```python
from build123d import *

# Parameters (mm, degrees)
SKETCH_1_W      = 2
SKETCH_1_H      = 12
EXTRUDE_1_DEPTH = 2.9
EXTRUDE_START   = -2
SKETCH_2_W      = 3.3
SKETCH_2_H      = 1.5
SKETCH_2_H_2    = 1.8
EXTRUDE_2_DEPTH = 5
SKETCH_3_W      = 10.525
SKETCH_3_H      = 2.9
EXTRUDE_3_DEPTH = 2
EXTRUDE_START_2 = -2.9
SKETCH_5_W      = 5
SKETCH_5_H      = 1
EXTRUDE_5_DEPTH = 17.8


with BuildPart() as part:
    # 草图1 → 凸台-拉伸1 (new body)
    with BuildSketch(Plane(origin=(0, 0, 0), x_dir=(1, 0, 0), z_dir=(0, 1, 0))):
        Rectangle(SKETCH_1_W, SKETCH_1_H)
    extrude(amount=EXTRUDE_1_DEPTH)

    # 草图2 → 凸台-拉伸2 (add)
    with BuildSketch(Plane(origin=(1, 0, 0), x_dir=(0, 0, -1), z_dir=(1, 0, 0)).offset(EXTRUDE_START)):
        with Locations((4.35, 3.25)):
            Rectangle(SKETCH_2_W, SKETCH_2_H)
        with Locations((4.35, -0.2)):
            Rectangle(SKETCH_2_W, SKETCH_2_H_2)
    extrude(amount=EXTRUDE_2_DEPTH)

    # 草图3 → 凸台-拉伸3 (add)
    with BuildSketch(Plane.ZY.offset(1)):
        with Locations((2.5625, 1.45)):
            Rectangle(SKETCH_3_W, SKETCH_3_H)
    extrude(amount=-EXTRUDE_3_DEPTH)

    # 草图5 → 凸台-拉伸5 (add)
    with BuildSketch(Plane(origin=(0, 2.9, 0), x_dir=(1, 0, 0), z_dir=(0, 1, 0)).offset(EXTRUDE_START_2)):
        with Locations((1.5, -7.325)):
            Rectangle(SKETCH_5_W, SKETCH_5_H)
        with Locations((1.5, -8.325)):
            Rectangle(SKETCH_5_W, SKETCH_5_H)
    extrude(amount=EXTRUDE_5_DEPTH)


solid = part.part
```
Can you work these out from the model? Positions are in its coordinate system, mm. A direction names the side the tool comes from. Coordinates: 2 decimals unless noted, no trailing zeros. Write each loop counter-clockwise with the first axis right and the second up, starting at its lowest first coordinate (ties: lowest second). Pieces come first, ordered by that corner, then holes. Notation, with made-up numbers: M 65,87 L 120,87 A19 cw 120,115 Z; hole C 63,-5.75 d6. An arc over 180 degrees is marked long. Write item = value, one per line. Start each with the question number.
Q1. If I drill on L1, parallel to Y at x = 2, z = -4; L2, parallel to Z at x = 2.8, y = 8.5 (3 decimals); L3, parallel to Y at x = 0, z = 2.25, over which ranges is the centre line in solid material (lowest first)? Write a range as [from, to].
Q2. I'm going to push flat-ended pins straight in: pin 1 (1.6 mm diameter, centred on x = 2.5, z = -3.5, fed in from +Y); pin 2 (0.9 mm diameter, centred on y = 2, z = 1.5, fed in from +X); pin 3 (8 mm diameter, centred on y = 3.5, z = 0, fed in from +X); pin 4 (1 mm diameter, centred on x = 0.5, z = 3.5, fed in from +Y). Where does each tip first touch, or does it pass through?
Q3. If we section it at A-A, the plane x = 1.75: Write out the boundary of the cut face in (y, z) (3 decimals), then the cut area to 3 significant figures.
Q4. If we section it at C-C, the plane x = 0.7: Write out the boundary of the cut face in (y, z) (3 decimals).
Q5. Thinking about a two-plate mould opening in Y: for faces 1 (the face through (2, 2.5, -4)), 2 (the face through (1, -1.1, -4)), 3 (the face through (0, 2.9, 2)), which applies, released by +Y, released by -Y, zero draft, split by the parting line, or undercut?
Q6. If we section it at B-B, the plane y = 3.5: Write out the boundary of the cut face in (x, z) (3 decimals), then the cut area to 3 significant figures.
Q7. If we section it at D-D, the plane z = -4.75: Write out the boundary of the cut face in (x, y), then the cut area to 3 significant figures.
Q8. On a 3-axis mill with a long thin cutter (end or side, diameter ignored), from which of +Z, -Z, +X, -X, +Y, -Y can I reach the whole of each face in a straight line? I mean faces 4 (the face through (1.5, -0.4, -2.7)), 5 (the face through (2, 0.7, -4)), 6 (the face through (1.5, 3.2, -2.7)), 7 (the face through (1, 4, -4)), 8 (the face through (0, 0, 3)). Say none if no direction works.
Check sheet entries:
q1.L1 = [-1.1, 0.7], [2.5, 4]
q1.L2 = [6.825, 8.825]
q1.L3 = [0, 2.9]
q2.pin_1 = 4
q2.pin_2 = 1
q2.pin_3 = 4
q2.pin_4 = 2.9
q3.outline = M -1.1,-6 L 0.7,-6 L 0.7,-2.7 L -1.1,-2.7 Z; M 0,6.825 L 17.8,6.825 L 17.8,8.825 L 0,8.825 Z; M 2.5,-6 L 4,-6 L 4,-2.7 L 2.5,-2.7 Z
q3.area = 46.5 mm²
q4.outline = M -1.1,-6 L 4,-6 L 4,-2.7 L 2.9,-2.7 L 2.9,6.825 L 17.8,6.825 L 17.8,8.825 L 0,8.825 L 0,-2.7 L -1.1,-2.7 Z
q5.face_1 = undercut
q5.face_2 = released by -Y
q5.face_3 = released by +Y
q6.outline = M -1,-6 L 4,-6 L 4,-2.7 L -1,-2.7 Z; M -1,6.825 L 4,6.825 L 4,8.825 L -1,8.825 Z
q6.area = 26.5 mm²
q7.outline = M -1,-1.1 L 4,-1.1 L 4,0.7 L 1,0.7 L 1,2.5 L 4,2.5 L 4,4 L -1,4 Z
q7.area = 20.1 mm²
q8.face_4 = +X, -Y
q8.face_5 = -Z, +X
q8.face_6 = +X, +Y
q8.face_7 = -Z, +X, -X, +Y
q8.face_8 = +Z, +X, -X, -Y
